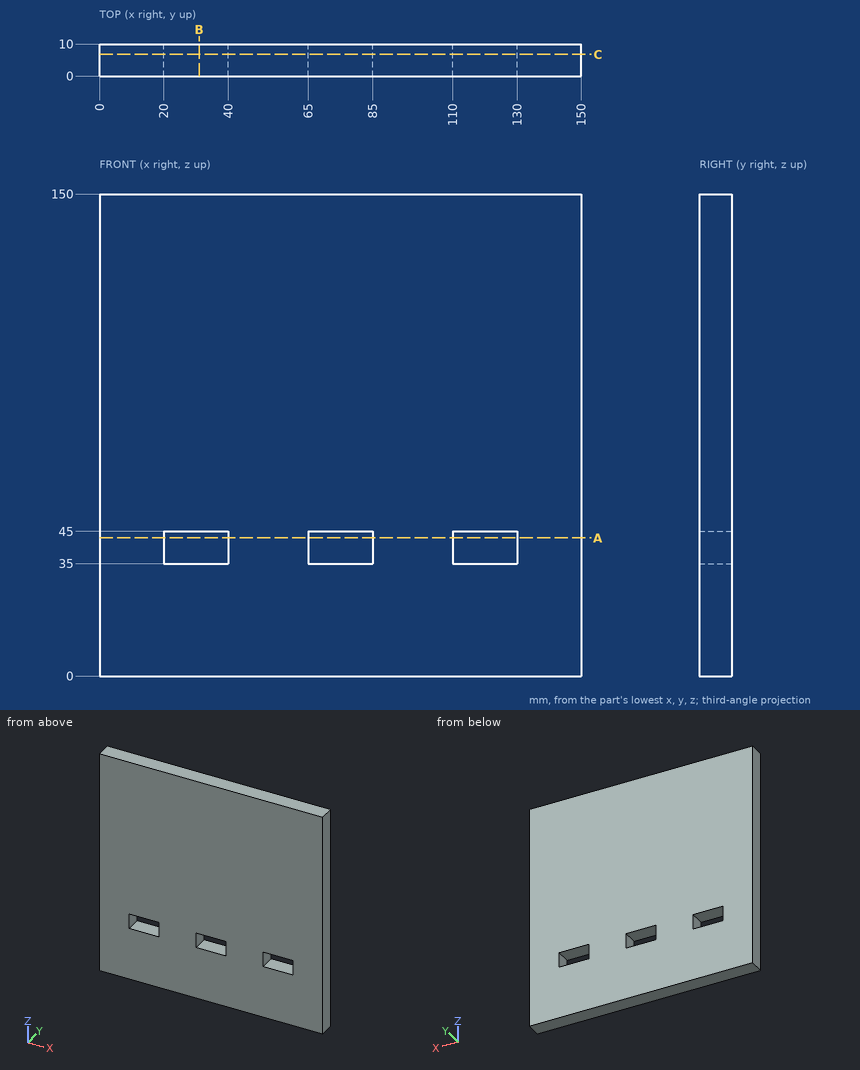
Part print with two shaded views. Sizes in mm from the minimum x, y, z corner. Round coordinates to 2 decimals unless told otherwise and drop trailing zeros. Order: outer loops, then holes, each group sorted by start corner. A loop starts at its lowest first (then second) coordinate and runs counter-clockwise, first axis right, second up. Notation, with made-up numbers: M -34,45.25 L 6,45.25 A13 ccw 6,56.25 Z; hole C -15.75,40 d10. An arc over 180 degrees is marked long. Use CSV: the item, a comma, the result in double quotes.
Item 1: Saw through at B-B (x = 31). List the corners of the cut face in (y, z).
Worked answers:
outline,"M 0,0 L 10,0 L 10,35 L 0,35 Z; M 0,45 L 10,45 L 10,150 L 0,150 Z"
Item 2: Saw through at C-C (y = 6.75). List the corners of the cut face in (x, z), plus the area to 3 significant figures.
Worked answers:
outline,"M 0,0 L 150,0 L 150,150 L 0,150 Z; hole M 20,35 L 40,35 L 40,45 L 20,45 Z; hole M 65,35 L 85,35 L 85,45 L 65,45 Z; hole M 110,35 L 130,35 L 130,45 L 110,45 Z"
area,"21,900 mm²"
Item 3: Saw through at A-A (z = 43). List the corners of the cut face in (x, y).
Worked answers:
outline,"M 0,0 L 20,0 L 20,10 L 0,10 Z; M 40,0 L 65,0 L 65,10 L 40,10 Z; M 85,0 L 110,0 L 110,10 L 85,10 Z; M 130,0 L 150,0 L 150,10 L 130,10 Z"
Item 4: Probe probe 1 along Z at (x, y) = (120.5, 4.75); probe 2 along X at (y, z) = (5, 43.5). List the from-to ranges inside material, lowest first.
Worked answers:
probe 1,"0 to 35, 45 to 150"
probe 2,"0 to 20, 40 to 65, 85 to 110, 130 to 150"
